The listing builds one solid part. Answer for the finished solid, in the listing's coordinates (mm). Face numbers are marked on the shaded views. Give positions to 0.01 mm unless a question says otherwise; leave off trailing zeros. Loops run counter-clockwise (first coordinate to the right, second up) from the corner with the lowest first, then second, coordinate; pieces in that order, holes last.
Item 1: Section D-D, the plane x = -23.5 is taken. Give the vertices of the cut face in (y, z), and give its area (3 significant figures).
Item 2: Section B-B, the plane y = -3 is taken. Give the vertices of the cut face in (x, z), and give its area (3 significant figures).
Item 3: Consider line 1 along Y through (x, z) = (-23, 1.75); line 2 along Y through (x, z) = (-20, 1.75); line 3 along X through (y, z) = (-4, 3.5). Determine where each line is inside the solid, lowest interval first.
Item 4: Section A-A, the plane x = -21.5 is taken. Give the vertices of the cut face in (y, z), and give its area (3 significant figures).
Item 5: The mould has two halves that part along Y. Classify the marked faces 1, 2, 3 and 4: pulls with the +Y half, pulls with the -Y half, needs draft (parallel to the pull), parting line crosses it, or undercut.
Item 6: Each of these flat-tipped pins is pushed along its axis until it touches: pin 1 Ø5 at (x, y) = (-21.77, -4.01) entering from +Z; pin 2 Ø4 at (x, y) = (-20, 24) entering from +Z. Where does it stop, or does it pass through?
Item 7: Section C-C, the plane z = 1 is taken. Give the vertices of the cut face in (x, y).
from build123d import *

# Parameters (mm, degrees)
F0_W     = 16
F0_H     = 48
F0_R     = 2.75
F1_DEPTH = 6
F2_R     = 4.25
F3_DEPTH = 3
F4_SIZE  = 1


with BuildPart() as f1:
    # F0 (on Top) → F1 (new body)
    with BuildSketch(Plane.XY):
        with Locations((-21.765074, 7.98561)):
            Rectangle(F0_W, F0_H)
        with Locations((-21.765074, -4.01439)):
            Circle(F0_R, mode=Mode.SUBTRACT)
        with Locations((-21.765074, 23.98561)):
            Circle(F0_R, mode=Mode.SUBTRACT)
    extrude(amount=F1_DEPTH)

    # F2 (on face) → F3 (cut)
    with BuildSketch(Plane.XY.offset(6)):
        with Locations((-21.765074, 23.98561)):
            Circle(F2_R)
        with Locations((-21.765074, -4.01439)):
            Circle(F2_R)
    extrude(amount=-F3_DEPTH, mode=Mode.SUBTRACT)

    # F4
    f4_edges = [f1.edges().sort_by_distance(p)[0] for p in [
        (-29.765074, 31.98561, 3),
        (-21.765074, 31.98561, 6),
        (-13.765074, 31.98561, 3),
        (-29.765074, 7.98561, 6),
        (-13.765074, 7.98561, 6),
    ]]
    chamfer(f4_edges, length=F4_SIZE)


solid = f1.part
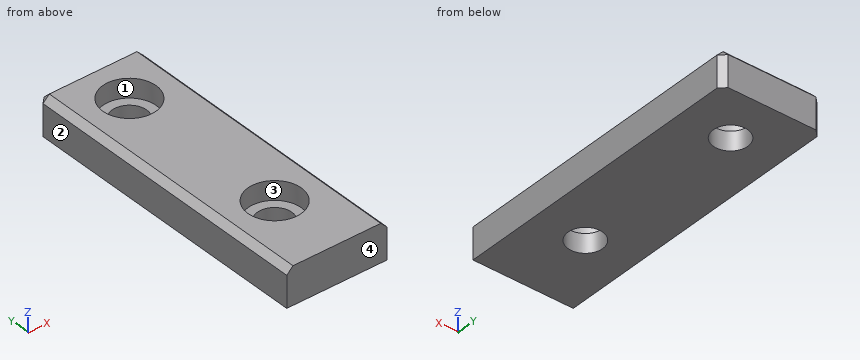
Worked answers:
1. outline: (-16.01, 0) - (-6.15, 0) - (-6.15, 3) - (-7.89, 3) - (-7.89, 6) - (-16.01, 6) - close; (-1.88, 0) - (21.85, 0) - (21.85, 3) - (20.11, 3) - (20.11, 6) - (-0.13, 6) - (-0.13, 3) - (-1.88, 3) - close; (26.12, 0) - (31.99, 0) - (31.99, 5) - (30.99, 6) - (27.87, 6) - (27.87, 3) - (26.12, 3) - close
1. area: 215 mm2
2. outline: (-29.77, 0) - (-24.32, 0) - (-24.32, 3) - (-25.89, 3) - (-25.89, 6) - (-28.77, 6) - (-29.77, 5) - close; (-19.21, 0) - (-13.77, 0) - (-13.77, 5) - (-14.77, 6) - (-17.64, 6) - (-17.64, 3) - (-19.21, 3) - close
2. area: 54.9 mm2
3. line 1: y = -16.01 to -6.47, -1.56 to 21.53, 26.44 to 31.99
3. line 2: y = -16.01 to -6.12, -1.91 to 21.88, 26.09 to 31.99
3. line 3: x = -29.77 to -26.02, -17.52 to -13.77
4. outline: (-16.01, 0) - (-6.75, 0) - (-6.75, 3) - (-8.26, 3) - (-8.26, 6) - (-16.01, 6) - close; (-1.28, 0) - (21.25, 0) - (21.25, 3) - (19.74, 3) - (19.74, 6) - (0.23, 6) - (0.23, 3) - (-1.28, 3) - close; (26.72, 0) - (31.99, 0) - (31.99, 5) - (30.99, 6) - (28.23, 6) - (28.23, 3) - (26.72, 3) - close
4. area: 204 mm2
5. face 1: undercut
5. face 2: needs draft
5. face 3: undercut
5. face 4: pulls with the -Y half
6. pin 1: passes through
6. pin 2: stops at z = 3
7. outline: (-29.77, -16.01) - (-13.77, -16.01) - (-13.77, 30.99) - (-14.77, 31.99) - (-28.77, 31.99) - (-29.77, 30.99) - close; hole circle Ø5.5 at (-21.77, -4.01); hole circle Ø5.5 at (-21.77, 23.99)
